Build history of the part. All positions in model axes, mm. Round coordinates to 2 decimals unless told otherwise and drop trailing zeros. Write each loop counter-clockwise with the first axis right and the second up, starting at its lowest first coordinate (ties: lowest second). Pieces come first, ordered by that corner, then holes. Notation, with made-up numbers: (14.25, -35) -> (63.25, -35) arc R33 cw to (63.25, 1) -> close; hole circle Ø5 at (-24.75, -32). An arc over 180 degrees is marked (long way). Answer as CSV lines item,"result".
Solid Edge part; units mm, degrees
sketch "Sketch1" plane through (0, 50.7, 0) normal (0, -1, 0) x (1, 0, 0)
  line L0 (21, 13.45) -> (-421, 13.45)
  line L1 (-421, 13.45) -> (-421, -13.45)
  line L2 (21, -13.45) -> (-421, -13.45)
  line L3 (21, -13.45) -> (21, 13.45)
  line L4 (-417, 9.45) -> (17, 9.45)
  line L5 (17, 9.45) -> (17, -9.45)
  line L6 (17, -9.45) -> (-417, -9.45)
  line L7 (-417, -9.45) -> (-417, 9.45)
extrude "Protrusion1" add sketch "Sketch1" against normal blind 5
sketch "Sketch2" plane through (0, 50.7, 0) normal (0, -1, 0) x (1, 0, 0)
  line L0 (-156, -9.45) -> (-156, 9.45)
  line L1 (-156, 9.45) -> (-160, 9.45)
  line L2 (-160, 9.45) -> (-160, -9.45)
  line L3 (-160, -9.45) -> (-156, -9.45)
  line L4 (-244, 9.45) -> (-244, -9.45)
  line L5 (-244, -9.45) -> (-240, -9.45)
  line L6 (-240, -9.45) -> (-240, 9.45)
  line L7 (-240, 9.45) -> (-244, 9.45)
extrude "ExtrudedProtrusion_2" add sketch "Sketch2" against normal blind 5
sketch "Sketch3" plane through (-200, 77.8, 0) normal (0, 1, 0) x (1, 0, 0)
  line L0 (-29, 2.3247) -> (-29, 7.3247)
  line L1 (-29, 7.3247) -> (-25, 7.3247)
  line L2 (-25, 7.3247) -> (-25, 2.3247)
  line L3 (-25, 2.3247) -> (-29, 2.3247)
  line L4 (-29, -12.6753) -> (-29, -7.6753)
  line L5 (-29, -7.6753) -> (-25, -7.6753)
  line L6 (-25, -7.6753) -> (-25, -12.6753)
  line L7 (-25, -12.6753) -> (-29, -12.6753)
  line L8 (29, -12.625) -> (25, -12.625)
  line L9 (25, -12.625) -> (25, -7.625)
  line L10 (25, -7.625) -> (29, -7.625)
  line L11 (29, -7.625) -> (29, -12.625)
  line L12 (25, 2.375) -> (25, 7.375)
  line L13 (25, 7.375) -> (29, 7.375)
  line L14 (29, 7.375) -> (29, 2.375)
  line L15 (29, 2.375) -> (25, 2.375)
extrude "ExtrudedProtrusion_3" add sketch "Sketch3" along normal blind 40
sketch "Sketch4" plane through (-229, 108.8, -7.375) normal (0.9545, 0.2964, 0.0339) x (0.2966, -0.955, 0)
  line L0 (-6.793, -0.4095) -> (-6.793, -4.4095)
  line L1 (-6.793, -4.4095) -> (-1.793, -4.4095)
  line L2 (-1.793, -4.4095) -> (-1.793, -0.4095)
  line L3 (-1.793, -0.4095) -> (-6.793, -0.4095)
extrude "ExtrudedProtrusion_6" add sketch "Sketch4" against normal blind 197.9 and the other way blind 2.75
sketch "Sketch5" plane through (-229, 108.8, 12.625) normal (0.955, 0.2966, -0.0046) x (0.2966, -0.955, 0)
  line L0 (-6.3917, 4.4374) -> (-6.3917, 0.4374)
  line L1 (-6.3917, 0.4374) -> (-1.3917, 0.4374)
  line L2 (-1.3917, 0.4374) -> (-1.3917, 4.4374)
  line L3 (-1.3917, 4.4374) -> (-6.3917, 4.4374)
extrude "ExtrudedProtrusion_8" add sketch "Sketch5" against normal blind 195.9 and the other way blind 2.3
mirror "Mirror1" about plane through (-200, 97.8, -4.8247) normal (1, 0, 0) of "ExtrudedProtrusion_6", "ExtrudedProtrusion_8"
sketch "Sketch6" plane through (-225, 97.8, -4.8247) normal (1, 0, 0) x (0, -1, 0)
  line L0 (-17.0981, -13.0124) -> (-12.3285, -13.0124)
  line L1 (-12.3285, -13.0124) -> (-12.3285, -17.0124)
  line L2 (-12.3285, -17.0124) -> (-17.0981, -17.0124)
  line L3 (-17.0981, -17.0124) -> (-17.0981, -13.0124)
  line L4 (-12.668, -1.8567) -> (-17.4833, -1.8567)
  line L5 (-17.4833, -1.8567) -> (-17.4833, 2.141)
  line L6 (-17.4833, 2.141) -> (-12.668, 2.141)
  line L7 (-12.668, 2.141) -> (-12.668, -1.8567)
extrude "Protrusion2" add sketch "Sketch6" along normal up to vertex (50 mm away)
properties material "Carbon Fiber"
1. Drop flat-ended pins along their axis: pin 1 Ø1 at (y, z) = (101.5, -2.5) entering from -X; pin 2 Ø3 at (x, y) = (-228, 98.5) entering from -Z; pin 3 Ø3 at (x, z) = (-134.5, -8) entering from +Y. Give the stop position or say it passes through.
Results found:
pin 1,"stops at x = -229"
pin 2,"stops at z = -7.32"
pin 3,"stops at y = 105.04"
2. Cut at B-B, the plane z = 3.75. Write the cut outline in (x, y), then the cut area to 3 significant figures.
Results found:
outline,"(-421, 50.7) -> (-417, 50.7) -> (-417, 55.7) -> (-421, 55.7) -> close; (-244, 50.7) -> (-240, 50.7) -> (-240, 55.7) -> (-244, 55.7) -> close; (-160, 50.7) -> (-156, 50.7) -> (-156, 55.7) -> (-160, 55.7) -> close; (17, 50.7) -> (21, 50.7) -> (21, 55.7) -> (17, 55.7) -> close"
area,"80.0 mm2"
3. Mould opens along X. For faces 1 (the flat face through (-322.167, 86.557, 10.599)), 2 (the flat face through (-321.436, 81.549, 10.659)), 3 (the flat face through (-199, 50.7, 10)), 4 (the flat face through (-78.564, 81.549, 10.603)) say: +X half, -X half, draft (parallel to the pull), parting line (faces both ways), or undercut.
Results found:
face 1,"-X half"
face 2,"undercut"
face 3,"draft"
face 4,"undercut"
4. Cut at C-C, the plane y = 88.5. Count the separate pieces of the cut face and the enclosed holes in it, then the cut area to 3 significant figures.
Results found:
separate pieces,"8"
enclosed holes,"0"
area,"350 mm2"
5. Probe line 1 along X through (y, z) = (78, 8.5); line 2 along Y through (x, z) = (-393, 10.25); line 3 along Y through (x, z) = (-45, 9.5). List the from-to ranges inside material, lowest first.
Results found:
line 1,"x = -229 to -225, -175 to -171"
line 2,"y = 50.7 to 55.7, 59.32 to 64.56"
line 3,"y = 50.7 to 55.7, 71.12 to 76.36"
6. Cut at A-A, the plane x = -211.5. Write the cut outline in (y, z).
Results found:
outline,"(50.7, -13.45) -> (55.7, -13.45) -> (55.7, -9.45) -> (50.7, -9.45) -> close; (50.7, 9.45) -> (55.7, 9.45) -> (55.7, 13.45) -> (50.7, 13.45) -> close; (110.13, 8.19) -> (114.9, 8.19) -> (114.9, 12.19) -> (110.13, 12.19) -> close; (110.47, -6.97) -> (115.28, -6.97) -> (115.28, -2.97) -> (110.47, -2.97) -> close"
